Here's how the part is built. I have some questions about the finished solid (model axes, mm). Coordinates: 2 decimals unless noted, no trailing zeros. Write each loop counter-clockwise with the first axis right and the second up, starting at its lowest first coordinate (ties: lowest second). Pieces come first, ordered by that corner, then holes. Notation, with made-up numbers: (32, 11) - (48, 11) arc R23 ccw to (48, 48) - close; hole circle Ø7 at (-36.75, 18.5). An arc over 180 degrees is marked (long way). Answer in a Markdown table with one row per item. Add a question column.
Item 1: Imagine slicing it at D-D (x = 107). Please give me the cut outline in (y, z).
Item 2: Imagine slicing it at C-C (z = 6). State how many separate pieces and enclosed holes the cut face has, plus the area to 3 significant figures.
Item 3: If I drill on probe 1 along X at (y, z) = (1, 6); probe 2 along Z at (x, y) = (144, 2); probe 3 along X at (y, z) = (33, 19), over which ranges is the centre line in solid material (lowest first)? Write a range as from..to.
Item 4: Imagine slicing it at A-A (x = 6). Please give me the cut outline in (y, z), plus the area to 4 significant figures.
Item 5: We'd pull the mould along X, two halves only. Please class faces 1 (the face through (134.4, 21.85, 34.59)), 2 (the face through (21, 13, 20)), 3 (the face through (139, 0, 20)), 4 (the face through (15, 18, 20)): +X half, -X half, draft (parallel to the pull), parting line (faces both ways), or undercut.
Item 6: Imagine slicing it at B-B (z = 13.5). Please give me the cut outline in (x, y), plus the area to 3 significant figures.
Item 7: I'm going to push flat-ended pins straight in: pin 1 (5 mm diameter, centred on x = 8, z = 10.5, fed in from +Y); pin 2 (9 mm diameter, centred on x = 83.5, z = 17.5, fed in from -Y); pin 3 (10 mm diameter, centred on x = 31.5, y = 35, fed in from +Z). Where does each tip first touch, or does it pass through?
from build123d import *

# Parameters (mm, degrees)
SKETCH_1_W          = 150
SKETCH_1_H          = 40
EXTRUDE_1_DEPTH     = 40
CUT_EXTRUDE_1_REACH = 162.312
SKETCH_2_W          = 15
SKETCH_2_H          = 35
CUT_EXTRUDE_2_REACH = 162.312
SKETCH_3_W          = 108
SKETCH_3_H          = 34
CUT_EXTRUDE_3_REACH = 148.373
SKETCH_5_R          = 2
CUT_EXTRUDE_4_DEPTH = 5
CHAMFER_1_SIZE      = 2.5
FILLET_2_R          = 2
FILLET_3_R          = 2


with BuildPart() as part:
    # 草图1 → 凸台-拉伸1 (new body)
    with BuildSketch(Plane.XY):
        with Locations((75, 20)):
            Rectangle(SKETCH_1_W, SKETCH_1_H)
    extrude(amount=EXTRUDE_1_DEPTH)

    # 草图2 → 切除-拉伸1 (cut, up to next)
    with BuildSketch(Plane(origin=(0, 0, 0), x_dir=(-1, 0, 0), z_dir=(0, 0, -1)), mode=Mode.PRIVATE) as cut_extrude_1_sk1:
        with Locations((-142.5, 22.5)):
            Rectangle(SKETCH_2_W, SKETCH_2_H)
    cut_extrude_1_tool1 = extrude(cut_extrude_1_sk1.sketch, amount=-CUT_EXTRUDE_1_REACH, mode=Mode.PRIVATE) & part.part
    # 草图2 → 切除-拉伸1 (cut, up to next)
    with BuildSketch(Plane(origin=(0, 0, 0), x_dir=(-1, 0, 0), z_dir=(0, 0, -1)), mode=Mode.PRIVATE) as cut_extrude_1_sk2:
        with Locations((-7.5, 22.5)):
            Rectangle(SKETCH_2_W, SKETCH_2_H)
    cut_extrude_1_tool2 = extrude(cut_extrude_1_sk2.sketch, amount=-CUT_EXTRUDE_1_REACH, mode=Mode.PRIVATE) & part.part
    add(cut_extrude_1_tool1.solids().sort_by_distance((142.5, 22.5, 0))[0], mode=Mode.SUBTRACT)
    add(cut_extrude_1_tool2.solids().sort_by_distance((7.5, 22.5, 0))[0], mode=Mode.SUBTRACT)

    # 草图3 → 切除-拉伸2 (cut, up to next)
    with BuildSketch(Plane(origin=(0, 0, 0), x_dir=(-1, 0, 0), z_dir=(0, 0, -1)), mode=Mode.PRIVATE) as cut_extrude_2_sk1:
        with Locations((-75, 17)):
            Rectangle(SKETCH_3_W, SKETCH_3_H)
    cut_extrude_2_tool1 = extrude(cut_extrude_2_sk1.sketch, amount=-CUT_EXTRUDE_2_REACH, mode=Mode.PRIVATE) & part.part
    add(cut_extrude_2_tool1.solids().sort_by_distance((75, 17, 0))[0], mode=Mode.SUBTRACT)

    # 切除-拉伸3: up to this face of the body (flat: up to its plane)
    cut_extrude_3_end = Plane(part.part.faces().sort_by_distance((15, 22.5, 20))[0])
    # 草图4 → 切除-拉伸3 (cut, up to the picked face)
    with BuildSketch(Plane(origin=(135, 0, 0), x_dir=(0, 0, -1), z_dir=(1, 0, 0)), mode=Mode.PRIVATE) as cut_extrude_3_sk1:
        Polygon((-40, 40), (-40, 5), (-30, 40), align=None)
    cut_extrude_3_tool1 = split(extrude(cut_extrude_3_sk1.sketch, amount=-CUT_EXTRUDE_3_REACH, mode=Mode.PRIVATE), bisect_by=cut_extrude_3_end, keep=Keep.BOTH, mode=Mode.PRIVATE)
    # 草图4 → 切除-拉伸3 (cut, up to the picked face)
    with BuildSketch(Plane(origin=(135, 0, 0), x_dir=(0, 0, -1), z_dir=(1, 0, 0)), mode=Mode.PRIVATE) as cut_extrude_3_sk2:
        Polygon((-10, 40), (0, 40), (0, 5), align=None)
    cut_extrude_3_tool2 = split(extrude(cut_extrude_3_sk2.sketch, amount=-CUT_EXTRUDE_3_REACH, mode=Mode.PRIVATE), bisect_by=cut_extrude_3_end, keep=Keep.BOTH, mode=Mode.PRIVATE)
    add(cut_extrude_3_tool1.solids().sort_by(Axis((135, 28.333333, 36.666667), (-1, 0, 0)))[0], mode=Mode.SUBTRACT)
    add(cut_extrude_3_tool2.solids().sort_by(Axis((135, 28.333333, 3.333333), (-1, 0, 0)))[0], mode=Mode.SUBTRACT)

    # 草图5 → 切除-拉伸4 (cut)
    with BuildSketch(Plane.XZ):
        with Locations(Location((6, 6, 0), (0, 0, 270))):
            Circle(SKETCH_5_R)
        with Locations(Location((6, 34, 0), (0, 0, 270))):
            Circle(SKETCH_5_R)
    cut_extrude_4 = extrude(amount=-CUT_EXTRUDE_4_DEPTH, mode=Mode.SUBTRACT)

    # 镜向5: 切除-拉伸4 across plane
    add(cut_extrude_4.mirror(Plane.ZY.offset(-75)), mode=Mode.SUBTRACT)

    # 倒角1
    chamfer_1_edges = [part.edges().sort_by_distance(p)[0] for p in [
        (144, 5, 36),
        (6, 5, 8),
        (6, 5, 36),
        (144, 5, 8),
    ]]
    chamfer(chamfer_1_edges, length=CHAMFER_1_SIZE)

    # 圆角2
    fillet_2_edges = [part.edges().sort_by_distance(p)[0] for p in [
        (135, 22.5, 5),
        (135, 40, 20),
        (135, 22.5, 35),
        (15, 22.5, 35),
        (15, 40, 20),
        (15, 22.5, 5),
        (75, 40, 10),
        (75, 40, 30),
        (21, 19.5, 4.142857143),
        (75, 34, 8.285714286),
        (129, 19.5, 4.142857143),
        (129, 19.5, 35.857142857),
        (21, 19.5, 35.857142857),
        (75, 34, 31.714285714),
    ]]
    fillet(fillet_2_edges, radius=FILLET_2_R)

    # 圆角3
    fillet_3_edges = [part.edges().sort_by_distance(p)[0] for p in [
        (150, 2.5, 40),
        (0, 2.5, 0),
        (0, 2.5, 40),
        (150, 2.5, 0),
    ]]
    fillet(fillet_3_edges, radius=FILLET_3_R)


solid = part.part
Here are the results:
| question | item | result |
|---|---|---|
| 1 | outline | (34, 10.94) arc R2 ccw to (36.55, 9.01) - (38.55, 9.59) arc R2 ccw to (40, 11.51) - (40, 28.49) arc R2 ccw to (38.55, 30.41) - (36.55, 30.99) arc R2 ccw to (34, 29.06) - close |
| 2 | separate pieces | 4 |
| 2 | enclosed holes | 0 |
| 2 | area | 397 mm2 |
| 3 | probe 1 | x = 0..4, 8..21, 129..142, 146..150 |
| 3 | probe 2 | z = 0..4, 8..32, 36..40 |
| 3 | probe 3 | x = 15..21, 129..135 |
| 4 | outline | (0, 0) - (5, 0) - (5, 1.5) - (2.5, 4) - (0, 4) - close; (0, 8) - (2.5, 8) - (5, 10.5) - (5, 29.5) - (2.5, 32) - (0, 32) - close; (0, 36) - (2.5, 36) - (5, 38.5) - (5, 40) - (0, 40) - close |
| 4 | area | 147.5 mm2 |
| 5 | face 1 | +X half |
| 5 | face 2 | undercut |
| 5 | face 3 | draft |
| 5 | face 4 | -X half |
| 6 | outline | (0, 0) - (21, 0) - (21, 34) - (129, 34) - (129, 0) - (150, 0) - (150, 5) - (135, 5) - (135, 38) arc R2 ccw to (133, 40) - (17, 40) arc R2 ccw to (15, 38) - (15, 5) - (0, 5) - close |
| 6 | area | 1,280 mm2 |
| 7 | pin 1 | stops at y = 5 |
| 7 | pin 2 | stops at y = 34 |
| 7 | pin 3 | stops at z = 31.06 |
